Read the model definition and answer for the solid it produces. Units are mm, in the model's axes. A direction names the side the tool comes from. Coordinates: 2 decimals unless noted, no trailing zeros. Order: outer loops, then holes, each group sorted by start corner. A loop starts at its lowest first (then second) coordinate and runs counter-clockwise, first axis right, second up. Notation, with made-up numbers: (-20.75, 42) - (13.25, 42) arc R21 cw to (13.25, 49) - close; hole circle Ø6 at (12.25, 29). An arc over 180 degrees is marked (long way). Use one line per item in the form item = value.
```python
from build123d import *

# Parameters (mm, degrees)
ESBO_O1_W                = 3
ESBO_O1_H                = 68
RESSALTO_EXTRUS_O1_DEPTH = 12
ESBO_O2_W                = 5
ESBO_O2_H                = 1.5
RESSALTO_EXTRUS_O2_DEPTH = 3


with BuildPart() as part:
    # Esboço1 → Ressalto-extrusão1 (new body)
    with BuildSketch(Plane(origin=(0, 0, 0), x_dir=(1, 0, 0), z_dir=(0, 1, 0))):
        Rectangle(ESBO_O1_W, ESBO_O1_H)
    extrude(amount=RESSALTO_EXTRUS_O1_DEPTH)

    # Esboço2 → Ressalto-extrusão2 (add)
    with BuildSketch(Plane(origin=(1.5, 0, 0), x_dir=(0, 0, -1), z_dir=(1, 0, 0))):
        with Locations((-18.5, -0.75)):
            Rectangle(ESBO_O2_W, ESBO_O2_H)
        with Locations((18.5, -0.75)):
            Rectangle(ESBO_O2_W, ESBO_O2_H)
    extrude(amount=-RESSALTO_EXTRUS_O2_DEPTH)


solid = part.part
```
(1) Section B-B, the plane z = 29 is taken. Write down the section's boundary in (x, y), then the cut area to 3 significant figures.
Answer list:
outline = (-1.5, 0) - (1.5, 0) - (1.5, 12) - (-1.5, 12) - close
area = 36.0 mm2
(2) Section A-A, the plane x = 0.45 is taken. Write down the section's boundary in (y, z), then the cut area to 3 significant figures.
Answer list:
outline = (-1.5, -21) - (0, -21) - (0, -34) - (12, -34) - (12, 34) - (0, 34) - (0, 21) - (-1.5, 21) - (-1.5, 16) - (0, 16) - (0, -16) - (-1.5, -16) - close
area = 831 mm2
(3) Which of the six approach directions +Z, -Z, +X, -X, +Y, -Y give full straight-line access (tool end or side, diameter ignored) to faces 4 (the flat face through (0, 0, -28)), 5 (the flat face through (0, 0, 0)), 6 (the flat face through (-1.5, 7, 0))?
Answer list:
face_4 = -Z, +X, -X, -Y
face_5 = +X, -X, -Y
face_6 = +Z, -Z, -X, +Y, -Y
(4) A straight line is drawn through the part: L1, parallel to Y at x = -0.85, z = 6.5. Find the intervals that lie inside material, in ascending order.
Answer list:
L1 = 0 to 12
(5) The mould has two halves that part along Z. Classify faces 1 (the flat face through (0, -1, 21)), 2 (the flat face through (0, 0, 27)), 3 (the flat face through (0, -1, -16)): +Z half, -Z half, draft (parallel to the pull), parting line (faces both ways), or undercut.
Answer list:
face_1 = +Z half
face_2 = draft
face_3 = undercut
(6) Given pin 1 Ø0.9 at (x, z) = (0, -29.5) entering from -Y; pin 2 Ø0.8 at (x, y) = (0.5, -0.5) entering from -Z; pin 3 Ø0.8 at (x, y) = (0.5, -1) entering from +Z, each flat-ended and moving along its own axis, determine where each tip first touches the part or whether it passes through.
Answer list:
pin_1 = 0
pin_2 = -21
pin_3 = 21
